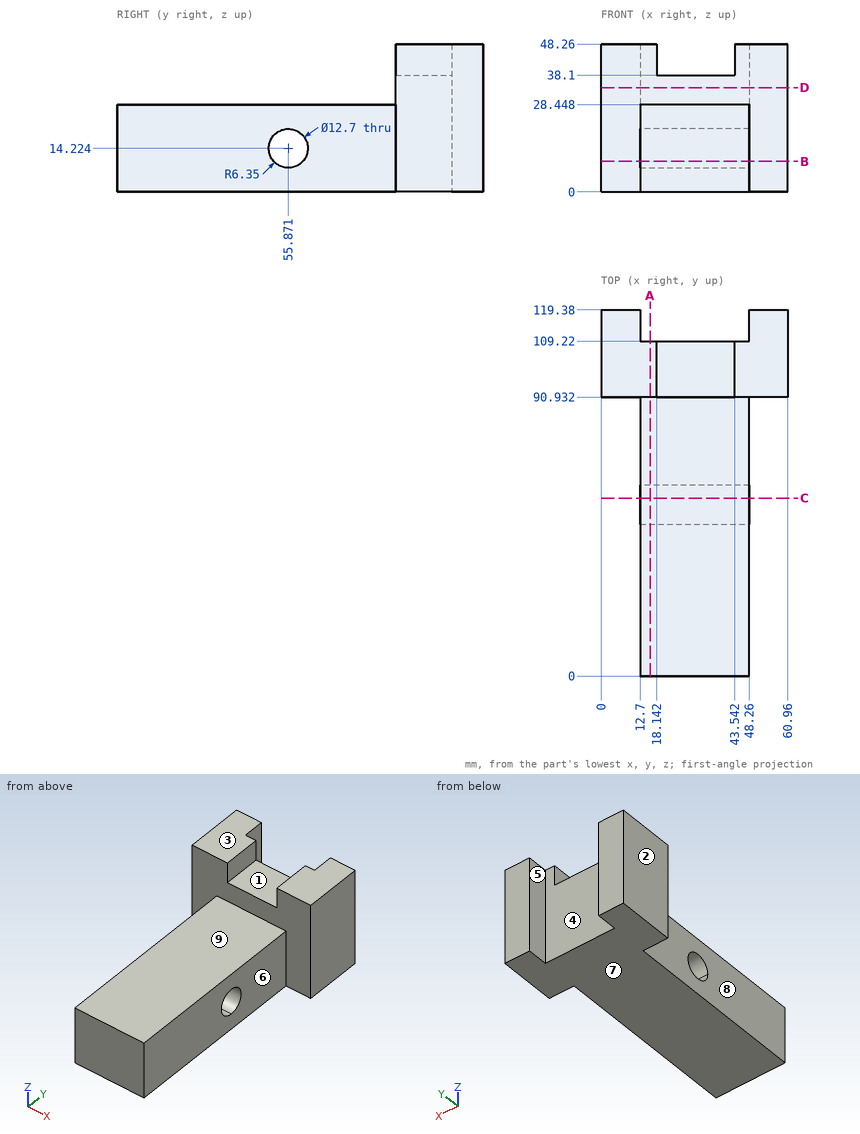
Here's the drawing with two shaded views (mm, measured from the low corner). I have some questions. A direction names the side the tool comes from. Give positions to 0.01 mm unless a question says otherwise; leave off trailing zeros. Write each loop counter-clockwise with the first axis right and the second up, starting at its lowest first coordinate (ties: lowest second). Pieces come first, ordered by that corner, then holes. Notation, with made-up numbers: (54, -9.5) - (58, -9.5) arc R9 ccw to (58, -4.5) - close; hole circle Ø2 at (22, -11.5). An arc over 180 degrees is marked (long way). Write item = value, one per line. Start each with the question number.
1. Thinking about a two-plate mould opening in X: for the marked faces 1, 2, 3 and 4, which applies, released by +X, released by -X, zero draft, split by the parting line, or undercut?
2. Imagine slicing it at B-B (z = 10). Please give me the cut outline in (x, y), and give its area (3 significant figures).
3. Imagine slicing it at A-A (x = 16). Please give me the cut outline in (y, z), and give its area (3 significant figures).
4. Please list where these lines run through material, in increasing order: line 1 (X direction, y = 114, z = 26); line 2 (Y direction, x = 15.5, z = 40.5); line 3 (Z direction, x = 42, y = 31).
5. Imagine slicing it at C-C (y = 58). Please give me the cut outline in (x, z), and give its area (3 significant figures).
6. Imagine slicing it at D-D (z = 34). Please give me the cut outline in (x, y).
7. On a 3-axis mill with a long thin cutter (end or side, diameter ignored), from which of +Z, -Z, +X, -X, +Y, -Y can I reach the whole of each face in a straight line? I mean the marked faces 5, 6, 7, 8 and 9. Say none if no direction works.
8. For pin 1 (23 mm diameter, centred on y = 25.5, z = 12, fed in from -X); pin 2 (8.5 mm diameter, centred on y = 40, z = 20, fed in from +X); pin 3 (9 mm diameter, centred on x = 28.5, y = 101.5, fed in from +Z), each with a flat end and sliding along its axis, tell me the tip position at first contact or that it passes through.
Worked answers:
q1.face_1 = undercut
q1.face_2 = released by -X
q1.face_3 = zero draft
q1.face_4 = undercut
q2.outline = (0, 90.93) - (12.7, 90.93) - (12.7, 60.61) - (48.26, 60.61) - (48.26, 90.93) - (60.96, 90.93) - (60.96, 119.38) - (48.26, 119.38) - (48.26, 109.22) - (12.7, 109.22) - (12.7, 119.38) - (0, 119.38) - close; (12.7, 0) - (48.26, 0) - (48.26, 51.13) - (12.7, 51.13) - close
q2.area = 4,270 mm2
q3.outline = (0, 0) - (109.22, 0) - (109.22, 48.26) - (90.93, 48.26) - (90.93, 28.45) - (0, 28.45) - close; hole (49.52, 14.22) arc R6.35 ccw to (55.87, 7.87) arc R6.35 ccw (long way) to start
q3.area = 3,340 mm2
q4.line_1 = 0 to 12.7, 48.26 to 60.96
q4.line_2 = 90.93 to 109.22
q4.line_3 = 0 to 28.45
q5.outline = (12.7, 0) - (48.26, 0) - (48.26, 8.24) - (12.7, 8.24) - close; (12.7, 20.21) - (48.26, 20.21) - (48.26, 28.45) - (12.7, 28.45) - close
q5.area = 586 mm2
q6.outline = (0, 90.93) - (60.96, 90.93) - (60.96, 119.38) - (48.26, 119.38) - (48.26, 109.22) - (12.7, 109.22) - (12.7, 119.38) - (0, 119.38) - close
q7.face_5 = +Z, -Z, +Y
q7.face_6 = +Z, -Z, +X, -Y
q7.face_7 = -Z, +X, -X, +Y, -Y
q7.face_8 = +Z, -Z, -X, -Y
q7.face_9 = +Z, +X, -X, -Y
q8.pin_1 = 12.7
q8.pin_2 = 48.26
q8.pin_3 = 38.1
